The model under review builds one solid part; all positions refer to its coordinate system, in mm. A direction names the side the tool comes from. Round coordinates to 2 decimals unless told otherwise and drop trailing zeros. Write each loop counter-clockwise with the first axis right and the second up, starting at its lowest first coordinate (ties: lowest second). Pieces come first, ordered by that corner, then holes. Notation, with made-up numbers: (39, 10) -> (47, 10) arc R17 cw to (47, 43) -> close; hole circle Ø10 at (-22.75, 7). An arc over 180 degrees is marked (long way). Use CSV: the item, a comma, the result in double quotes. Start each with the question number.
1) Mouldability with a two-part tool opening along X and no side actions: class faces 3 (the face through (-1.4, -1.52, 3.29)), 4 (the face through (0.02, -7.41, 2.62)), 5 (the face through (1.15, -8, 6)) as released by +X, released by -X, zero draft, split by the parting line, or undercut.
2) Machinability: for faces 1 (the face through (-0.016, 11.029, 10.067)), 2 (the face through (-2, 2, 6.5)), which of the approach directions +Z, -Z, +X, -X, +Y, -Y give a long, thin tool a straight path to every point of the face, cutting with its end or side? Answer none if there is none.
3) Take a section at C-C, the plane z = 7.75. Give the boundary of the cut face in (x, y), then the cut area to 3 significant figures.
4) Take a section at A-A, the plane x = 0. Give the boundary of the cut face in (y, z) (3 decimals).
5) For pin 1 Ø4.5 at (y, z) = (7.5, 5) entering from +X; pin 2 Ø3 at (x, y) = (-1.5, -6.5) entering from -Z; pin 3 Ø2 at (x, y) = (0, 0.5) entering from +Z; pin 4 Ø4 at (x, z) = (0, 5) entering from -Y, all flat-tipped, find the tip position at first contact; note any pin that passes through.
6) Take a section at B-B, the plane y = 0. Give the boundary of the cut face in (x, z) (3 decimals).
7) Take a section at D-D, the plane z = 2.5. Give the boundary of the cut face in (x, y) (3 decimals).
8) Wall thickness on probe 1 along X at (y, z) = (4.75, 4.75); probe 2 along Y at (x, z) = (0.25, 9); probe 3 along Z at (x, y) = (0.5, 2.5): over which ranges is each line inside the solid? List them lowest first. Write a range as [from, to].
from build123d import *

# Parameters (mm, degrees)
PAD_DEPTH = 1.15


with BuildPart() as pad:
    # Sketch001 → Pad (new body, symmetric)
    with BuildSketch(Plane.YZ):
        with BuildLine():
            Line((2.5, 0), (2.5, 6.5))
            Line((2.5, 6.5), (4, 6.5))
            Line((4, 6.5), (6.050198, 9.559301))
            ThreePointArc((10.730567, 5.173209), (10.972336, 10.121439), (6.050198, 9.559301))
            Line((4, 0), (10.730567, 5.173209))
            Line((2.5, 0), (4, 0))
        make_face()
        with BuildLine():
            Line((-10.730567, 5.173209), (-4, 0))
            Line((-4, 0), (-2.5, 0))
            Line((-2.5, 0), (-2.5, 6.5))
            Line((-2.5, 6.5), (-4, 6.5))
            Line((-4, 6.5), (-6.050198, 9.559301))
            ThreePointArc((-6.050198, 9.559301), (-10.972336, 10.121439), (-10.730567, 5.173209))
        make_face()
    extrude(amount=PAD_DEPTH, both=True)


with BuildPart() as obj1:
    # Sketch → Revolution (revolve)
    with BuildSketch(Plane.YZ):
        Polygon((2.5, 0), (2.065, 0.251147), (2.065, 6.248853), (2.5, 6.5), (3.5, 6.5), (4, 0), align=None)
    revolve(axis=Axis((0, 0, 0), (0, 0, 1)))

    # Fusion: union Pad
    add(pad.part)


solid = obj1.part
Values found:
1,face 3,"undercut"
1,face 4,"zero draft"
1,face 5,"released by +X"
2,face 1,"+X, -X"
2,face 2,"+Z, +X, -X"
3,outline,"(-1.15, -12) -> (1.15, -12) -> (1.15, -4.84) -> (-1.15, -4.84) -> close; (-1.15, 4.84) -> (1.15, 4.84) -> (1.15, 12) -> (-1.15, 12) -> close"
3,area,"32.9 mm²"
4,outline,"(-10.731, 5.173) -> (-4, 0) -> (-2.5, 0) -> (-2.065, 0.251) -> (-2.065, 6.249) -> (-2.5, 6.5) -> (-4, 6.5) -> (-6.05, 9.559) arc R3.25 ccw (long way) to start; (2.065, 0.251) -> (2.5, 0) -> (4, 0) -> (10.731, 5.173) arc R3.25 ccw (long way) to (6.05, 9.559) -> (4, 6.5) -> (2.5, 6.5) -> (2.065, 6.249) -> close"
5,pin 1,"x = 1.15"
5,pin 2,"z = 0.8"
5,pin 3,"through"
5,pin 4,"y = -11.91"
6,outline,"(-4, 0) -> (-2.5, 0) -> (-2.065, 0.251) -> (-2.065, 6.249) -> (-2.5, 6.5) -> (-3.5, 6.5) -> close; (2.065, 0.251) -> (2.5, 0) -> (4, 0) -> (3.5, 6.5) -> (2.5, 6.5) -> (2.065, 6.249) -> close"
7,outline,"(-1.15, -7.253) -> (1.15, -7.253) -> (1.15, -3.63) arc R3.808 ccw to (1.15, 3.63) -> (1.15, 7.253) -> (-1.15, 7.253) -> (-1.15, 3.63) arc R3.808 ccw to (-1.15, -3.63) -> close; hole circle Ø4.13 at (0, 0)"
8,probe 1,"[-1.15, 1.15]"
8,probe 2,"[-11.75, -5.68], [5.68, 11.75]"
8,probe 3,"[0, 6.5]"
